Geometry: final body of the model. Coordinates: model frame, mm. A direction names the side the tool comes from. Give positions to 0.01 mm unless a question says otherwise; leave off trailing zeros. Loops run counter-clockwise (first coordinate to the right, second up) from the corner with the lowest first, then second, coordinate; pieces in that order, holes last.
from build123d import *

# Parameters (mm, degrees)
SKETCH1_W               = 33.02
SKETCH1_H               = 106.68
BOSS_EXTRUDE1_DEPTH     = 3.175
SKETCH3_W               = 3.175
SKETCH3_H               = 10.16
BOSS_EXTRUDE2_DEPTH     = 3.175
LPATTERN1_COUNT         = 5
LPATTERN1_PITCH         = 17.78
MIRROR1_COPY_1_SKETCH_W = 3.175
MIRROR1_COPY_1_SKETCH_H = 10.16
MIRROR1_COPY_1_DEPTH    = 3.175
MIRROR1_COPY_2_SKETCH_W = 3.175
MIRROR1_COPY_2_SKETCH_H = 10.16
MIRROR1_COPY_2_DEPTH    = 3.175
MIRROR1_COPY_3_SKETCH_W = 3.175
MIRROR1_COPY_3_SKETCH_H = 10.16
MIRROR1_COPY_3_DEPTH    = 3.175
MIRROR1_COPY_4_SKETCH_W = 3.175
MIRROR1_COPY_4_SKETCH_H = 10.16
MIRROR1_COPY_4_DEPTH    = 3.175
SKETCH4_W               = 3.175
SKETCH4_H               = 10.16
BOSS_EXTRUDE3_DEPTH     = 3.175
MIRROR3_COPY_1_SKETCH_W = 3.175
MIRROR3_COPY_1_SKETCH_H = 10.16
MIRROR3_COPY_1_DEPTH    = 3.175


with BuildPart() as part:
    # Sketch1 → Boss-Extrude1 (new body)
    with BuildSketch(Plane(origin=(0, 0, 0), x_dir=(0, 0, -1), z_dir=(1, 0, 0))):
        with Locations((0.241329403, -2.63343568)):
            Rectangle(SKETCH1_W, SKETCH1_H)
        with BuildLine():
            Line((4.051329403, 39.27656432), (-3.568670597, 39.27656432))
            ThreePointArc((-3.568670597, 39.27656432), (-8.95682427, 37.044717993), (-11.188670597, 31.65656432))
            Line((-11.188670597, 31.65656432), (-11.188670597, -36.92343568))
            ThreePointArc((-11.188670597, -36.92343568), (-8.95682427, -42.311589352), (-3.568670597, -44.54343568))
            Line((-3.568670597, -44.54343568), (4.051329403, -44.54343568))
            ThreePointArc((4.051329403, -44.54343568), (9.439483075, -42.311589352), (11.671329403, -36.92343568))
            Line((11.671329403, -36.92343568), (11.671329403, 31.65656432))
            ThreePointArc((11.671329403, 31.65656432), (9.439483075, 37.044717993), (4.051329403, 39.27656432))
        make_face(mode=Mode.SUBTRACT)
    extrude(amount=BOSS_EXTRUDE1_DEPTH)

    # Sketch3 → Boss-Extrude2 (add)
    with BuildSketch(Plane.XY.offset(16.268670597)):
        with Locations((1.5875, 32.92656432)):
            Rectangle(SKETCH3_W, SKETCH3_H)
    boss_extrude2 = extrude(amount=BOSS_EXTRUDE2_DEPTH)

    # LPattern1: Boss-Extrude2 ×5
    with Locations(*[(0, -i * LPATTERN1_PITCH, 0) for i in range(1, LPATTERN1_COUNT)]):
        add(boss_extrude2)

    # Mirror1: Boss-Extrude2 across plane
    add(boss_extrude2.mirror(Plane(origin=(0, 0, -0.241329403), x_dir=(1, 0, 0), z_dir=(0, 0, -1))))

    # Mirror1 copy 1 sketch → Mirror1 copy 1 (add)
    with BuildSketch(Plane(origin=(0, -17.78, -16.751329403), x_dir=(1, 0, 0), z_dir=(0, 0, -1))):
        with Locations((1.5875, -32.92656432)):
            Rectangle(MIRROR1_COPY_1_SKETCH_W, MIRROR1_COPY_1_SKETCH_H)
    extrude(amount=MIRROR1_COPY_1_DEPTH)

    # Mirror1 copy 2 sketch → Mirror1 copy 2 (add)
    with BuildSketch(Plane(origin=(0, -35.56, -16.751329403), x_dir=(1, 0, 0), z_dir=(0, 0, -1))):
        with Locations((1.5875, -32.92656432)):
            Rectangle(MIRROR1_COPY_2_SKETCH_W, MIRROR1_COPY_2_SKETCH_H)
    extrude(amount=MIRROR1_COPY_2_DEPTH)

    # Mirror1 copy 3 sketch → Mirror1 copy 3 (add)
    with BuildSketch(Plane(origin=(0, -53.34, -16.751329403), x_dir=(1, 0, 0), z_dir=(0, 0, -1))):
        with Locations((1.5875, -32.92656432)):
            Rectangle(MIRROR1_COPY_3_SKETCH_W, MIRROR1_COPY_3_SKETCH_H)
    extrude(amount=MIRROR1_COPY_3_DEPTH)

    # Mirror1 copy 4 sketch → Mirror1 copy 4 (add)
    with BuildSketch(Plane(origin=(0, -71.12, -16.751329403), x_dir=(1, 0, 0), z_dir=(0, 0, -1))):
        with Locations((1.5875, -32.92656432)):
            Rectangle(MIRROR1_COPY_4_SKETCH_W, MIRROR1_COPY_4_SKETCH_H)
    extrude(amount=MIRROR1_COPY_4_DEPTH)

    # Sketch4 → Boss-Extrude3 (add)
    with BuildSketch(Plane(origin=(0, 50.70656432, 0), x_dir=(1, 0, 0), z_dir=(0, 1, 0))):
        with Locations((1.5875, -7.378670597)):
            Rectangle(SKETCH4_W, SKETCH4_H)
    boss_extrude3 = extrude(amount=BOSS_EXTRUDE3_DEPTH)

    # Mirror2: Boss-Extrude3 across plane
    add(boss_extrude3.mirror(Plane(origin=(0, 0, -0.241329403), x_dir=(1, 0, 0), z_dir=(0, 0, -1))))

    # Mirror3: Boss-Extrude3 across plane
    add(boss_extrude3.mirror(Plane.ZX.offset(-2.63343568)))

    # Mirror3 copy 1 sketch → Mirror3 copy 1 (add)
    with BuildSketch(Plane(origin=(0, -55.97343568, -0.482658805), x_dir=(1, 0, 0), z_dir=(0, -1, 0))):
        with Locations((1.5875, -7.378670597)):
            Rectangle(MIRROR3_COPY_1_SKETCH_W, MIRROR3_COPY_1_SKETCH_H)
    extrude(amount=MIRROR3_COPY_1_DEPTH)


solid = part.part
Item 1: Draft query along Y for faces 5 (the face through (1.57, -42.25, 9.02)), 6 (the face through (2, -58, -2.781)), 7 (the face through (2, -59.148, -8)). Return one class per face: +Y half, -Y half, draft (parallel to the pull), parting line (faces both ways), or undercut.
Values follow:
face 5: undercut
face 6: draft
face 7: -Y half
Item 2: Set-up query: faces 1 (the face through (2, 27.847, -18)), 2 (the face through (2, -55.973, 14)), 3 (the face through (2, 20.227, 18)), 4 (the face through (2, 52, -12.941)). Return all of +Z, -Z, +X, -X, +Y, -Y with unobstructed straight access to the full face (end or side cutting, diameter ignored); none if empty.
Values follow:
face 1: -Z, +X, -X
face 2: +Z, +X, -X, -Y
face 3: +Z, +X, -X
face 4: -Z, +X, -X, +Y
Item 3: Pin query (flat end, axial travel): pin 1 (1 mm diameter, centred on x = 1, z = 17.5, fed in from -Y); pin 2 (1 mm diameter, centred on x = 1.5, z = -18.5, fed in from +Y); pin 3 (1.6 mm diameter, centred on x = 1, z = 17, fed in from -Y). Return the tip coordinate at first contact, or that it passes through.
Values follow:
pin 1: stops at y = -43.27
pin 2: stops at y = 38.01
pin 3: stops at y = -55.97
Item 4: Ray query, probe 1 along Y at (x, z) = (2.8, -17); probe 2 along Z at (x, y) = (1.75, 7); probe 3 along Y at (x, z) = (1.4, 4). Return the intervals inside material, ascending.
Values follow:
probe 1: y = -43.27 to -33.11, -25.49 to -15.33, -7.71 to 2.45, 10.07 to 20.23, 27.85 to 38.01
probe 2: z = -16.75 to -11.67, 11.19 to 16.27
probe 3: y = -59.15 to -44.53, 39.26 to 53.88
Item 5: Section query A-A on y = -24.5. Return loops of the section in (x, z) (3 decimals).
Values follow:
outline: (0, -19.926) - (3.175, -19.926) - (3.175, -11.671) - (0, -11.671) - close; (0, 11.189) - (3.175, 11.189) - (3.175, 19.444) - (0, 19.444) - close
Item 6: Section query B-B on z = -5.5. Return loops of the section in (x, y) (3 decimals).
Values follow:
outline: (0, -59.148) - (3.175, -59.148) - (3.175, -44.404) - (0, -44.404) - close; (0, 39.138) - (3.175, 39.138) - (3.175, 53.882) - (0, 53.882) - close
Item 7: Section query C-C on z = -14.5. Return loops of the section in (x, y) (3 decimals), plus the area to 3 significant figures.
Values follow:
outline: (0, -55.973) - (3.175, -55.973) - (3.175, 50.707) - (0, 50.707) - close
area: 339 mm2
